Drawing for the job (mm, zero at the part's lowest x, y, z). Coordinates: 2 decimals unless noted, no trailing zeros. Write each loop counter-clockwise with the first axis right and the second up, starting at its lowest first coordinate (ties: lowest second). Pieces come first, ordered by that corner, then holes. Notation, with made-up numbers: (34.5, 11.5) -> (90.5, 11.5) arc R7 ccw to (90.5, 23.5) -> close; hole circle Ø2 at (-29.75, 79). An arc over 180 degrees is marked (long way). Answer as CSV lines item,"result".
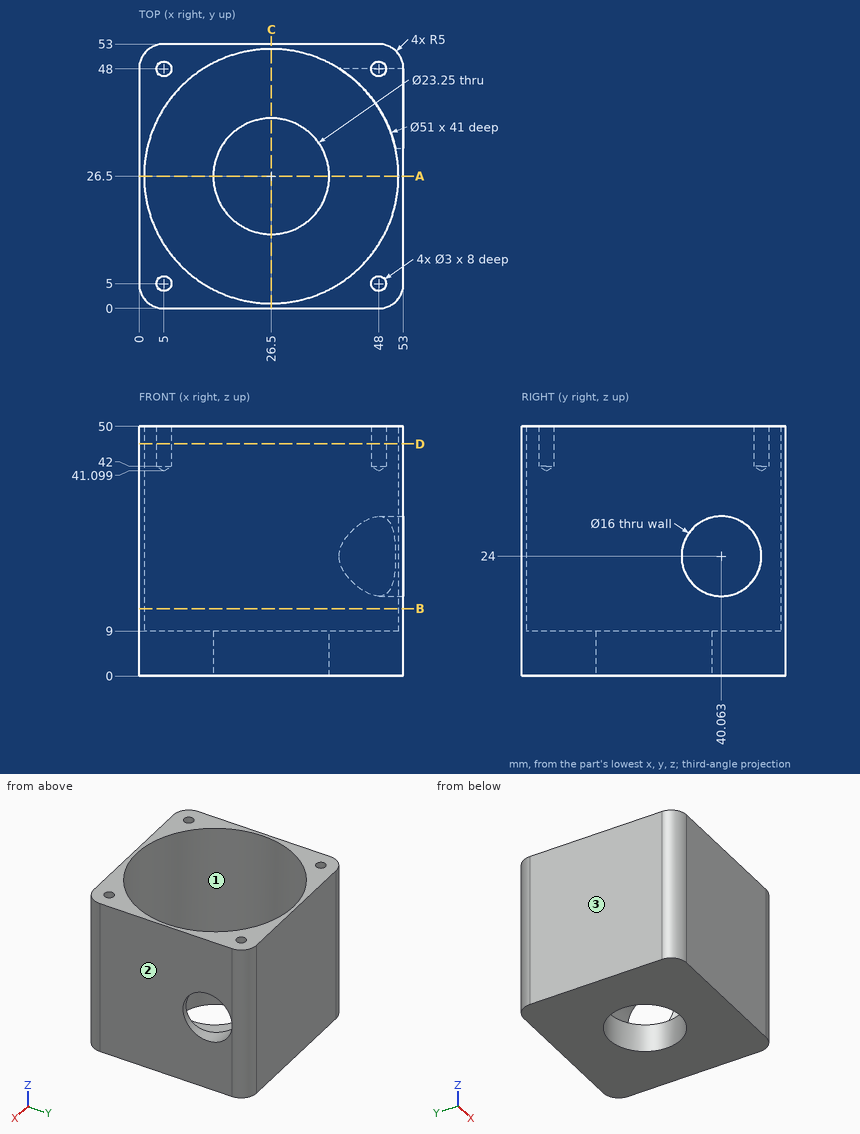
Item 1: Flat gauge pins, fed straight in: pin 1 (4 mm diameter, centred on x = 5, y = 5, fed in from +Z); pin 2 (2.5 mm diameter, centred on x = 5, y = 48, fed in from +Z); pin 3 (15.5 mm diameter, centred on x = 20, y = 22.5, fed in from +Z). Where does each tip first touch, or does it go through?
Answer below:
pin 1,"stops at z = 50"
pin 2,"stops at z = 41.85"
pin 3,"stops at z = 9"
Item 2: Two-plate mould, pull along X, no slides. Class the marked faces 1, 2 and 3: pulls with the +X half, pulls with the -X half, needs draft (parallel to the pull), parting line crosses it, or undercut.
Answer below:
face 1,"undercut"
face 2,"pulls with the +X half"
face 3,"pulls with the -X half"
Item 3: Saw through at D-D on z = 46.5. Give the cut face in (x, y).
Answer below:
outline,"(0, 5) arc R5 ccw to (5, 0) -> (48, 0) arc R5 ccw to (53, 5) -> (53, 48) arc R5 ccw to (48, 53) -> (5, 53) arc R5 ccw to (0, 48) -> close; hole circle Ø51 at (26.5, 26.5); hole circle Ø3 at (5, 5); hole circle Ø3 at (5, 48); hole circle Ø3 at (48, 5); hole circle Ø3 at (48, 48)"
Item 4: Saw through at A-A on y = 26.5. Give the cut face in (x, z) (1 decimal).
Answer below:
outline,"(0, 0) -> (14.9, 0) -> (14.9, 9) -> (1, 9) -> (1, 50) -> (0, 50) -> close; (38.1, 0) -> (53, 0) -> (53, 50) -> (52, 50) -> (52, 9) -> (38.1, 9) -> close"
Item 5: Wall check: line 1 (X direction, y = 48, z = 44); line 2 (Y direction, x = 48.5, z = 47.5) (1 decimal). Give the ranges that are in metal, low to high. Write a range as from..to.
Answer below:
line 1,"x = 0..3.5, 6.5..12.79, 40.21..46.5, 49.5..53"
line 2,"y = 0..3.6, 6.4..13.6, 39.4..46.6, 49.4..53"
Item 6: Saw through at B-B on z = 13.5. Give the cut face in (x, y), and give its area (3 significant figures).
Answer below:
outline,"(0, 5) arc R5 ccw to (5, 0) -> (48, 0) arc R5 ccw to (53, 5) -> (53, 48) arc R5 ccw to (48, 53) -> (5, 53) arc R5 ccw to (0, 48) -> close; hole circle Ø51 at (26.5, 26.5)"
area,"745 mm2"
